Check sheet for the modelled part. Datum: model origin and axes. Units: mm. Face numbers are marked on the shaded views. Give positions to 0.01 mm unless a question says otherwise; leave off trailing zeros. Order: outer loops, then holes, each group sorted by start corner. A loop starts at its lowest first (then second) coordinate and runs counter-clockwise, first axis right, second up.
Item 1: Sectioned sample at C-C on z = -138. Record the boundary of the cut face in (x, y).
Item 2: Sectioned sample at A-A on x = 64. Record the boundary of the cut face in (y, z), and give its area (3 significant figures).
Item 3: Gauge pin test, flat ends, axial feed: P1, Ø5, axis at x = 62, y = -10.5, coming from the +Z side; P2, Ø2, axis at x = 102, z = -216.5, coming from the -Y side; P3, Ø5, axis at x = 10, y = -24, coming from the +Z side; P4, Ø1.3, axis at x = 155, y = 1.5, coming from the -Z side. Record the tip position at first contact, or that the pin passes through.
Item 4: Release check for a two-part mould opening along Z. For the marked faces 1, 2 and 3 record: released by +Z, released by -Z, zero draft, split by the parting line, or undercut.
Item 5: Sectioned sample at B-B on y = -5.5. Record the boundary of the cut face in (x, z).
Item 6: Material ranges on line 1 along X through (y, z) = (-24, -2.2); line 2 along Z through (x, y) = (74, 2.5); line 3 along X through (y, z) = (-4, -132.5), recorded low to high.
Item 7: Sectioned sample at D-D on z = -201.5. Record the boundary of the cut face in (x, y).
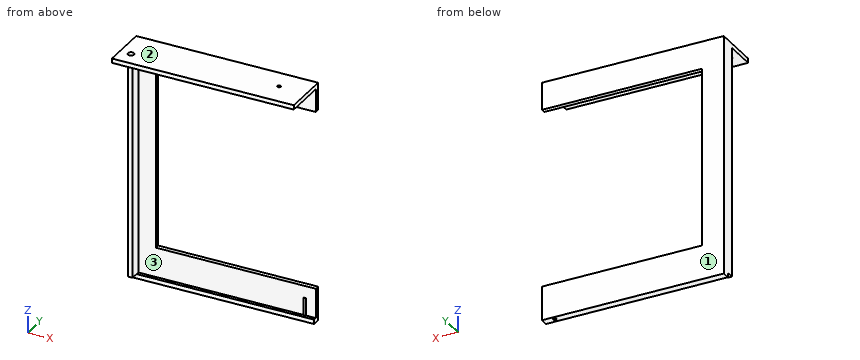
from build123d import *

# Parameters (mm, degrees)
SKETCH_1_W           = 165.5
SKETCH_1_H           = 38
EXTRUDE_1_DEPTH      = 4
SKETCH_2_W           = 20
SKETCH_2_H           = 215
EXTRUDE_2_DEPTH      = 4
SKETCH_3_W           = 211
SKETCH_3_H           = 10
EXTRUDE_3_DEPTH      = 4
SKETCH_4_W           = 145.5
SKETCH_4_H           = 25
EXTRUDE_4_DEPTH      = 4
SKETCH_5_R           = 1.5
CUT_EXTRUDE_1_DEPTH  = 4
SKETCH_6_W           = 165.5
SKETCH_6_H           = 7
EXTRUDE_5_DEPTH      = 4
SKETCH_7_W           = 145.5
SKETCH_7_H           = 27
EXTRUDE_6_DEPTH      = 4
SKETCH_8_R           = 2.75
CUT_EXTRUDE_2_DEPTH  = 4
MIRROR_START         = -4
MIRROR_3_OUTLINE_W   = 165.5
MIRROR_3_OUTLINE_H   = 42
MIRROR_3_OUTLINE_R   = 1.5
MIRROR_3_OUTLINE_R_2 = 2.75
MIRROR_3_DEPTH       = 4
MIRROR_START_2       = -215
MIRROR_3_2_DEPTH     = 211
MIRROR_START_3       = -25
MIRROR_3_3_OUTLINE_W = 145.5
MIRROR_3_3_OUTLINE_H = 4
MIRROR_3_3_DEPTH     = 21
MIRROR_START_4       = -219
MIRROR_3_4_OUTLINE_W = 165.5
MIRROR_3_4_OUTLINE_H = 7
MIRROR_3_4_DEPTH     = 4
SKETCH_9_W           = 186.740400525
SKETCH_9_H           = 237.71944978
CUT_EXTRUDE_3_DEPTH  = 278.696326947
SKETCH_10_W          = 145.5
SKETCH_10_H          = 27
EXTRUDE_7_DEPTH      = 4
SKETCH_11_R          = 1.5
CUT_EXTRUDE_4_DEPTH  = 20


# Read off the part's stored shape, not the designer's step: 镜向3
with BuildPart() as part:
    # 草图1 → 凸台-拉伸1 (new body)
    with BuildSketch(Plane.XY):
        with Locations((82.75, -19)):
            Rectangle(SKETCH_1_W, SKETCH_1_H)
    extrude(amount=EXTRUDE_1_DEPTH)

    # 草图2 → 凸台-拉伸2 (add)
    with BuildSketch(Plane(origin=(0, 0, 0), x_dir=(1, 0, 0), z_dir=(0, 1, 0))):
        with Locations((10, -107.5)):
            Rectangle(SKETCH_2_W, SKETCH_2_H)
    extrude(amount=EXTRUDE_2_DEPTH)

    # 草图3 → 凸台-拉伸3 (add)
    with BuildSketch(Plane.ZY):
        with Locations((109.5, -5)):
            Rectangle(SKETCH_3_W, SKETCH_3_H)
    extrude(amount=-EXTRUDE_3_DEPTH)

    # 草图4 → 凸台-拉伸4 (add)
    with BuildSketch(Plane(origin=(0, 0, 0), x_dir=(1, 0, 0), z_dir=(0, 1, 0))):
        with Locations((92.75, -12.5)):
            Rectangle(SKETCH_4_W, SKETCH_4_H)
    extrude(amount=EXTRUDE_4_DEPTH)

    # 草图5 → 切除-拉伸1 (cut)
    with BuildSketch(Plane(origin=(0, 0, 0), x_dir=(-1, 0, 0), z_dir=(0, 0, -1))):
        with Locations((-140.5, -16)):
            Circle(SKETCH_5_R)
    extrude(amount=-CUT_EXTRUDE_1_DEPTH, mode=Mode.SUBTRACT)

    # 草图6 → 凸台-拉伸5 (add)
    with BuildSketch(Plane.XY.offset(215)):
        with Locations((82.75, 0.5)):
            Rectangle(SKETCH_6_W, SKETCH_6_H)
    extrude(amount=EXTRUDE_5_DEPTH)

    # 草图8 → 切除-拉伸2 (cut)
    with BuildSketch(Plane(origin=(0, 0, 0), x_dir=(-1, 0, 0), z_dir=(0, 0, -1))):
        with Locations((-10, -24)):
            Circle(SKETCH_8_R)
    extrude(amount=-CUT_EXTRUDE_2_DEPTH, mode=Mode.SUBTRACT)

    # 镜向3 outline → 镜向3 (add)
    with BuildSketch(Plane.XY.offset(MIRROR_START)):
        with Locations((82.75, -17)):
            Rectangle(MIRROR_3_OUTLINE_W, MIRROR_3_OUTLINE_H)
        with Locations((140.5, -16)):
            Circle(MIRROR_3_OUTLINE_R, mode=Mode.SUBTRACT)
        with Locations((10, -24)):
            Circle(MIRROR_3_OUTLINE_R_2, mode=Mode.SUBTRACT)
    extrude(amount=MIRROR_3_DEPTH)

    # Mirror 3 2 outline → Mirror 3 2 (add)
    with BuildSketch(Plane.XY.offset(MIRROR_START_2)):
        Polygon((20, 0), (20, 4), (0, 4), (0, -10), (4, -10), (4, 0), align=None)
    extrude(amount=MIRROR_3_2_DEPTH)

    # Mirror 3 3 outline → Mirror 3 3 (add)
    with BuildSketch(Plane.XY.offset(MIRROR_START_3)):
        with Locations((92.75, 2)):
            Rectangle(MIRROR_3_3_OUTLINE_W, MIRROR_3_3_OUTLINE_H)
    extrude(amount=MIRROR_3_3_DEPTH)

    # Mirror 3 4 outline → Mirror 3 4 (add)
    with BuildSketch(Plane.XY.offset(MIRROR_START_4)):
        with Locations((82.75, 0.5)):
            Rectangle(MIRROR_3_4_OUTLINE_W, MIRROR_3_4_OUTLINE_H)
    extrude(amount=MIRROR_3_4_DEPTH)


with BuildPart() as body_2:
    # 草图7 → 凸台-拉伸6 (new body)
    with BuildSketch(Plane(origin=(0, 4, 0), x_dir=(1, 0, 0), z_dir=(0, 1, 0))):
        with Locations((92.75, -201.5)):
            Rectangle(SKETCH_7_W, SKETCH_7_H)
    extrude(amount=-EXTRUDE_6_DEPTH)


with BuildPart() as cut_extrude_3_tool:
    # 草图9 → 切除-拉伸3 (new, through all)
    with BuildSketch(Plane(origin=(0, 4, 0), x_dir=(1, 0, 0), z_dir=(0, 1, 0))):
        with Locations((93.370200263, -118.85972489)):
            Rectangle(SKETCH_9_W, SKETCH_9_H)
    extrude(amount=-CUT_EXTRUDE_3_DEPTH)


with BuildPart() as part_1:
    add(part.part)

    # 切除-拉伸3: cut by cut_extrude_3_tool
    add(cut_extrude_3_tool.part, mode=Mode.SUBTRACT)

    # 草图10 → 凸台-拉伸7 (add)
    with BuildSketch(Plane(origin=(0, 4, 0), x_dir=(1, 0, 0), z_dir=(0, 1, 0))):
        with Locations((92.75, 201.5)):
            Rectangle(SKETCH_10_W, SKETCH_10_H)
    extrude(amount=-EXTRUDE_7_DEPTH)

    # 草图11 → 切除-拉伸4 (cut)
    with BuildSketch(Plane(origin=(0, 0, -219), x_dir=(-1, 0, 0), z_dir=(0, 0, -1))):
        with Locations((-155.5, 1)):
            Circle(SKETCH_11_R)
    extrude(amount=-CUT_EXTRUDE_4_DEPTH, mode=Mode.SUBTRACT)


with BuildPart() as body_2_1:
    add(body_2.part)

    # 切除-拉伸3: cut by cut_extrude_3_tool
    add(cut_extrude_3_tool.part, mode=Mode.SUBTRACT)


solid = part_1.part
Report:
1. outline: (0, -10) - (4, -10) - (4, 0) - (20, 0) - (20, 4) - (0, 4) - close
2. outline: (-38, -4) - (0, -4) - (0, -25) - (4, -25) - (4, 0) - (-38, 0) - close; (-3, -219) - (4, -219) - (4, -188) - (0, -188) - (0, -215) - (-3, -215) - close
2. area: 388 mm2
3. P1: stops at z = 0
3. P2: stops at y = -3
3. P3: passes through
3. P4: stops at z = -199
4. face 1: zero draft
4. face 2: released by +Z
4. face 3: undercut
5. outline: (0, -215) - (4, -215) - (4, -4) - (165.5, -4) - (165.5, 0) - (0, 0) - close
6. line 1: x = 0 to 7.25, 12.75 to 165.5
6. line 2: z = -219 to -188, -25 to 0
6. line 3: x = 0 to 4
7. outline: (0, -10) - (4, -10) - (4, 0) - (154.38, 0) arc R1.5 cw (long way) to (156.62, 0) - (165.5, 0) - (165.5, 4) - (0, 4) - close
